Job drawing, mm, ordinate dimensions from the low corner. One solid piece. Give positions to 0.01 mm unless a question says otherwise; leave off trailing zeros. Write each loop counter-clockwise with the first axis right and the second up, starting at its lowest first coordinate (ties: lowest second). Pieces come first, ordered by that corner, then holes. Notation, with made-up numbers: (48.25, -7) - (79.25, -7) arc R22 ccw to (79.25, 12) - close; hole circle Ø1 at (37.5, 81.5). An arc over 180 degrees is marked (long way). Use a Markdown table: item, result. Add a question column.
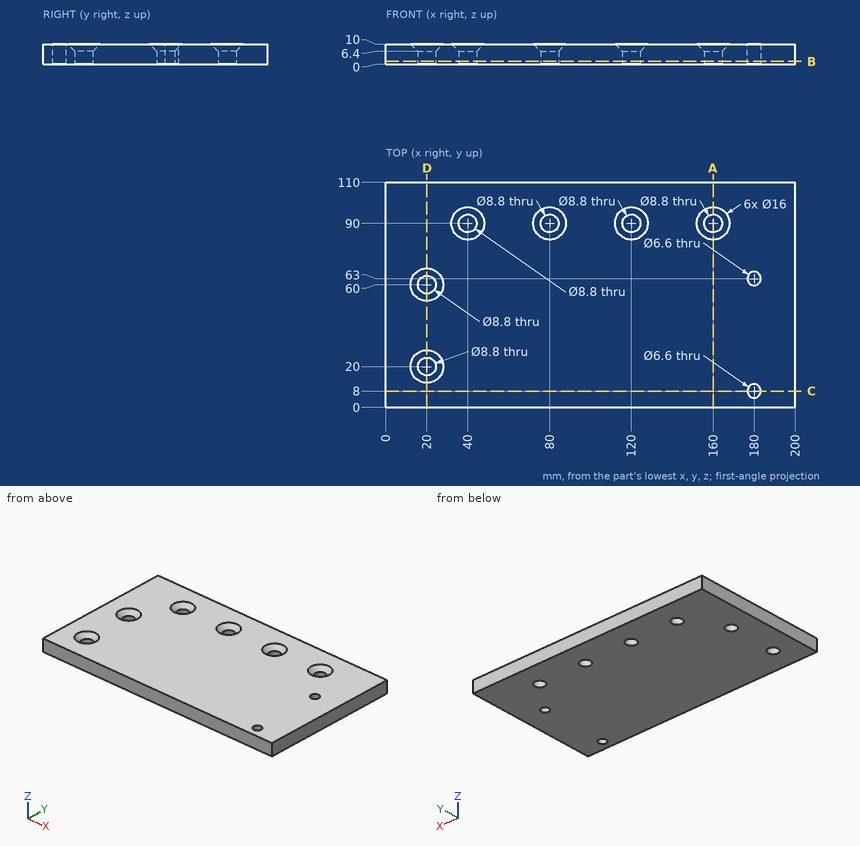
(1) Flat gauge pins, fed straight in: pin 1 (10 mm diameter, centred on x = 20, y = 20, fed in from +Z); pin 2 (5.5 mm diameter, centred on x = 40, y = 90, fed in from +Z). Where does each tip first touch, or does it go through?
(2) Band-saw the part on A-A (x = 160). Write the cut outline in (y, z), then the cut area to 3 significant figures.
(3) Probe probe 1 along X at (y, z) = (90, 4); probe 2 along Y at (x, z) = (20, 2.75); probe 3 along Y at (x, z) = (180, 7). List the from-to ranges inside material, lowest first. Write a range as [from, to].
(4) Band-saw the part on C-C (y = 8). Write the cut outline in (x, z).
(5) Band-saw the part on B-B (z = 1.5). Give the number of separate pieces and of enclosed holes in the cut face, then the cut area to 3 significant figures.
(6) Band-saw the part on D-D (x = 20). Write the cut outline in (y, z).
Model answer:
| question | item | result |
|---|---|---|
| 1 | pin 1 | stops at z = 7 |
| 1 | pin 2 | passes through |
| 2 | outline | (0, 0) - (85.6, 0) - (85.6, 6.4) - (82, 10) - (0, 10) - close; (94.4, 0) - (110, 0) - (110, 10) - (98, 10) - (94.4, 6.4) - close |
| 2 | area | 999 mm^2 |
| 3 | probe 1 | x = [0, 35.6], [44.4, 75.6], [84.4, 115.6], [124.4, 155.6], [164.4, 200] |
| 3 | probe 2 | y = [0, 15.6], [24.4, 55.6], [64.4, 110] |
| 3 | probe 3 | y = [0, 4.7], [11.3, 59.7], [66.3, 110] |
| 4 | outline | (0, 0) - (176.7, 0) - (176.7, 10) - (0, 10) - close; (183.3, 0) - (200, 0) - (200, 10) - (183.3, 10) - close |
| 5 | separate pieces | 1 |
| 5 | enclosed holes | 8 |
| 5 | area | 21,600 mm^2 |
| 6 | outline | (0, 0) - (15.6, 0) - (15.6, 6.4) - (12, 10) - (0, 10) - close; (24.4, 0) - (55.6, 0) - (55.6, 6.4) - (52, 10) - (28, 10) - (24.4, 6.4) - close; (64.4, 0) - (110, 0) - (110, 10) - (68, 10) - (64.4, 6.4) - close |
